Model file for the job. Use its own axes, mm. A direction names the side the tool comes from. Give positions to 0.01 mm unless a question says otherwise; leave off trailing zeros. Loops run counter-clockwise (first coordinate to the right, second up) from the corner with the lowest first, then second, coordinate; pieces in that order, holes last. Notation, with made-up numbers: M -11,-32.75 L 35,-32.75 A20 cw 35,-26.75 Z; hole C 63.25,46 d7. An arc over 180 degrees is marked long. Answer in a Markdown table with one row per item.
```python
from build123d import *

# Parameters (mm, degrees)
SKETCH_1_R      = 1.75
EXTRUDE_1_DEPTH = 2
SKETCH_3_W      = 8
SKETCH_3_H      = 6.75
SKETCH_3_R      = 1.75
SKETCH_3_H_2    = 6.25
SKETCH_3_W_2    = 8.45
EXTRUDE_2_DEPTH = 3


with BuildPart() as part:
    # 草图1 → 凸台-拉伸1 (new body)
    with BuildSketch(Plane.XY):
        Polygon((85.5, 49.25), (77.05, 49.25), (77.05, 6.25), (85.5, 6.25), (85.5, 0), (0, 0), (0, 55.5), (85.5, 55.5), align=None)
        with Locations((3.95, 51.05)):
            Circle(SKETCH_1_R, mode=Mode.SUBTRACT)
        with Locations((81.55, 51.05)):
            Circle(SKETCH_1_R, mode=Mode.SUBTRACT)
        with Locations((3.95, 4.45)):
            Circle(SKETCH_1_R, mode=Mode.SUBTRACT)
        with Locations((81.55, 4.45)):
            Circle(SKETCH_1_R, mode=Mode.SUBTRACT)
    extrude(amount=EXTRUDE_1_DEPTH)

    # 草图3 → 凸台-拉伸2 (add)
    # profile 1 of 4: a face of its own
    with BuildSketch(Plane.XY.offset(2)):
        with Locations((4, 52.125)):
            Rectangle(SKETCH_3_W, SKETCH_3_H)
        with Locations((3.95, 51.05)):
            Circle(SKETCH_3_R, mode=Mode.SUBTRACT)
    # profile 2 of 4: a face of its own
    with BuildSketch(Plane.XY.offset(2)):
        with Locations((4, 3.125)):
            Rectangle(SKETCH_3_W, SKETCH_3_H_2)
        with Locations((3.95, 4.45)):
            Circle(SKETCH_3_R, mode=Mode.SUBTRACT)
    # profile 3 of 4: a face of its own
    with BuildSketch(Plane.XY.offset(2)):
        with Locations((81.275, 52.375)):
            Rectangle(SKETCH_3_W_2, SKETCH_3_H_2)
        with Locations((81.55, 51.05)):
            Circle(SKETCH_3_R, mode=Mode.SUBTRACT)
    # profile 4 of 4: a face of its own
    with BuildSketch(Plane.XY.offset(2)):
        with Locations((81.275, 3.125)):
            Rectangle(SKETCH_3_W_2, SKETCH_3_H_2)
        with Locations((81.55, 4.45)):
            Circle(SKETCH_3_R, mode=Mode.SUBTRACT)
    extrude(amount=EXTRUDE_2_DEPTH)


solid = part.part
```
Q1. Probe probe 1 along Z at (x, y) = (73, 52); probe 2 along X at (y, z) = (5.5, 2.8); probe 3 along X at (y, z) = (32, 1.8). List the from-to ranges inside material, lowest first.
Reported:
| item | result |
|---|---|
| probe 1 | 0 to 2 |
| probe 2 | 0 to 2.55, 5.35 to 8, 77.05 to 80.15, 82.95 to 85.5 |
| probe 3 | 0 to 77.05 |
Q2. Saw through at C-C (x = 51.5). Give the cut face in (y, z).
Reported:
| item | result |
|---|---|
| outline | M 0,0 L 55.5,0 L 55.5,2 L 0,2 Z |
Q3. 3-axis set-ups, long thin cutter, end or side, ignore diameter. For faces 1 (the face through (81.17, 2.74, 2.46)), 2 (the face through (4, 2, 5)), 3 (the face through (8, 52, 3)), 4 (the face through (82.2, 6.25, 2.5)), 5 (the face through (5, 6.25, 3)): which of +Z, -Z, +X, -X, +Y, -Y reach the whole face in a straight line?
Reported:
| item | result |
|---|---|
| face 1 | +Z, -Z |
| face 2 | +Z, +X, -X, +Y, -Y |
| face 3 | +Z, +Y, -Y |
| face 4 | +Z, -Z, +X |
| face 5 | +Z, +X, -X |
Q4. Mould opens along X. For faces 6 (the face through (80, 49.25, 2)), 7 (the face through (77.05, 3, 3)), 8 (the face through (85.5, 52, 2)) say: released by +X, released by -X, zero draft, split by the parting line, or undercut.
Reported:
| item | result |
|---|---|
| face 6 | zero draft |
| face 7 | undercut |
| face 8 | released by +X |
Q5. Saw through at D-D (y = 21.5). Give the cut face in (x, z), and give its area (3 significant figures).
Reported:
| item | result |
|---|---|
| outline | M 0,0 L 77.05,0 L 77.05,2 L 0,2 Z |
| area | 154 mm² |
Q6. Drop flat-ended pins along their axis: pin 1 (2 mm diameter, centred on y = 46, z = 4.5, fed in from -X); pin 2 (1 mm diameter, centred on y = 22, z = 1, fed in from +X). Give the stop position or say it passes through.
Reported:
| item | result |
|---|---|
| pin 1 | through |
| pin 2 | x = 77.05 |
Q7. Saw through at A-A (z = 2.75). Give the cut face in (x, y).
Reported:
| item | result |
|---|---|
| outline | M 0,0 L 8,0 L 8,6.25 L 0,6.25 Z; M 0,48.75 L 8,48.75 L 8,55.5 L 0,55.5 Z; M 77.05,0 L 85.5,0 L 85.5,6.25 L 77.05,6.25 Z; M 77.05,49.25 L 85.5,49.25 L 85.5,55.5 L 77.05,55.5 Z; hole C 3.95,4.45 d3.5; hole C 3.95,51.05 d3.5; hole C 81.55,4.45 d3.5; hole C 81.55,51.05 d3.5 |
Q8. Saw through at B-B (y = 4.45). Give the cut face in (x, z).
Reported:
| item | result |
|---|---|
| outline | M 0,0 L 2.2,0 L 2.2,5 L 0,5 Z; M 5.7,0 L 79.8,0 L 79.8,5 L 77.05,5 L 77.05,2 L 8,2 L 8,5 L 5.7,5 Z; M 83.3,0 L 85.5,0 L 85.5,5 L 83.3,5 Z |
